For this review, use the dimensioned drawing (mm, ordinates from the lowest corner) and the shaded views. Coordinates: 2 decimals unless noted, no trailing zeros. Loops run counter-clockwise (first coordinate to the right, second up) from the corner with the lowest first, then second, coordinate; pieces in that order, holes last. Notation, with made-up numbers: (4.25, 18.25) - (57.25, 18.25) arc R22 cw to (57.25, 35.25) - close; hole circle Ø7 at (-32.75, 20). An arc over 180 degrees is marked (long way). Use one line per item in the form item = value. Start each with the question number.
(1) Add section A-A (y = 5.5). State the section outline as (x, z) points, plus the area to 3 significant figures.
(2) Add section B-B (z = 217.5). State the section outline as (x, y) points.
(3) For L1, parallel to X at y = 9, z = 135.5, list the stretches that pass through material, from the lowest coordinate up.
(4) Clearance check with flat-ended pins moving along their axes: pin 1 Ø8 at (x, z) = (1939, 173) entering from -Y; pin 2 Ø4 at (y, z) = (8, 374.5) entering from -X; pin 3 Ø6.5 at (y, z) = (9.5, 4.5) entering from +X; pin 4 Ø6.5 at (x, y) = (2194.5, 3.5) entering from +Z. State where each tip first meets the part, or that it passes through.
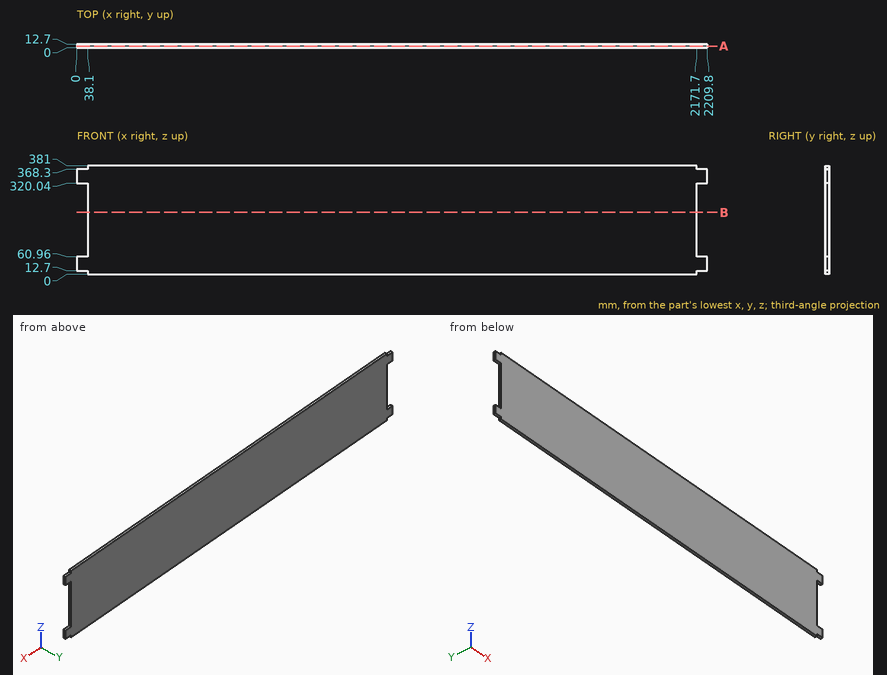
Computed values:
q1.outline = (0, 12.7) - (38.1, 12.7) - (38.1, 0) - (2171.7, 0) - (2171.7, 12.7) - (2209.8, 12.7) - (2209.8, 60.96) - (2171.7, 60.96) - (2171.7, 320.04) - (2209.8, 320.04) - (2209.8, 368.3) - (2171.7, 368.3) - (2171.7, 381) - (38.1, 381) - (38.1, 368.3) - (0, 368.3) - (0, 320.04) - (38.1, 320.04) - (38.1, 60.96) - (0, 60.96) - close
q1.area = 820,000 mm^2
q2.outline = (38.1, 0) - (2171.7, 0) - (2171.7, 12.7) - (38.1, 12.7) - close
q3.L1 = 38.1 to 2171.7
q4.pin_1 = 0
q4.pin_2 = 38.1
q4.pin_3 = 2171.7
q4.pin_4 = 368.3
